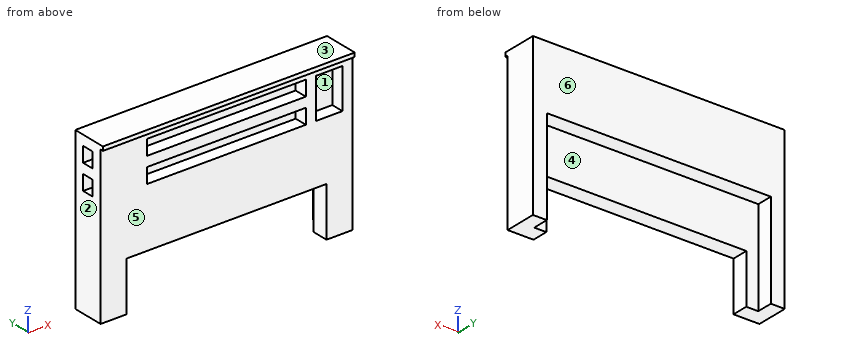
from build123d import *

# Parameters (mm, degrees)
F0_W     = 1016
F0_H     = 96.8375
F0_W_2   = 1611.3125
F0_H_2   = 25.4
F0_W_3   = 170.65625
F0_H_3   = 257.175
F1_DEPTH = 223.8375
F2_DEPTH = 101.6
F3_DEPTH = 19.05
F4_W     = 77.7875
F4_H     = 96.8375
F5_DEPTH = 190.5
F7_DEPTH = 101.6


with BuildPart() as f1:
    # F0 (on Front) → F1 (new body)
    with BuildSketch(Plane.XZ):
        Polygon((0, 698.5), (0, 0), (165.89375, 0), (165.89375, 317.5), (1445.41875, 317.5), (1445.41875, 0), (1611.3125, 0), (1611.3125, 698.5), (1547.8125, 698.5), (1377.15625, 698.5), (1313.65625, 698.5), (297.65625, 698.5), align=None)
        Polygon((0, 993.775), (0, 698.5), (297.65625, 698.5), (297.65625, 795.3375), (1313.65625, 795.3375), (1313.65625, 698.5), (1377.15625, 698.5), (1377.15625, 955.675), (1547.8125, 955.675), (1547.8125, 698.5), (1611.3125, 698.5), (1611.3125, 993.775), align=None)
        with Locations((805.65625, 907.25625)):
            Rectangle(F0_W, F0_H, mode=Mode.SUBTRACT)
        with Locations((805.65625, 746.91875)):
            Rectangle(F0_W, F0_H)
        with Locations((805.65625, 907.25625)):
            Rectangle(F0_W, F0_H)
        with Locations((805.65625, 1006.475)):
            Rectangle(F0_W_2, F0_H_2)
        with Locations((1462.484375, 827.0875)):
            Rectangle(F0_W_3, F0_H_3)
    extrude(amount=-F1_DEPTH)

    # F0 (on Front) → F2 (cut)
    with BuildSketch(Plane.XZ):
        with Locations((805.65625, 907.25625)):
            Rectangle(F0_W, F0_H)
        with Locations((805.65625, 746.91875)):
            Rectangle(F0_W, F0_H)
        with Locations((1462.484375, 827.0875)):
            Rectangle(F0_W_3, F0_H_3)
    extrude(amount=-F2_DEPTH, mode=Mode.SUBTRACT)

    # F0 (on Front) → F3 (cut)
    with BuildSketch(Plane.XZ):
        Polygon((0, 698.5), (0, 0), (165.89375, 0), (165.89375, 317.5), (1445.41875, 317.5), (1445.41875, 0), (1611.3125, 0), (1611.3125, 698.5), (1547.8125, 698.5), (1377.15625, 698.5), (1313.65625, 698.5), (297.65625, 698.5), align=None)
        Polygon((0, 993.775), (0, 698.5), (297.65625, 698.5), (297.65625, 795.3375), (1313.65625, 795.3375), (1313.65625, 698.5), (1377.15625, 698.5), (1377.15625, 955.675), (1547.8125, 955.675), (1547.8125, 698.5), (1611.3125, 698.5), (1611.3125, 993.775), align=None)
        with Locations((805.65625, 907.25625)):
            Rectangle(F0_W, F0_H, mode=Mode.SUBTRACT)
    extrude(amount=-F3_DEPTH, mode=Mode.SUBTRACT)

    # F4 (on face) → F5 (cut)
    with BuildSketch(Plane(origin=(0, 0, 0), x_dir=(0, -1, 0), z_dir=(-1, 0, 0))):
        with Locations((-121.44375, 907.25625)):
            Rectangle(F4_W, F4_H)
        with Locations((-121.44375, 746.91875)):
            Rectangle(F4_W, F4_H)
    extrude(amount=-F5_DEPTH, mode=Mode.SUBTRACT)

    # F6 (on face) → F7 (cut)
    with BuildSketch(Plane(origin=(0, 223.8375, 0), x_dir=(-1, 0, 0), z_dir=(0, 1, 0))):
        Polygon((-1522.4125, 609.6), (-1522.4125, 0), (-1445.41875, 0), (-1445.41875, 317.5), (-165.89375, 317.5), (-165.89375, 0), (-88.9, 0), (-88.9, 609.6), align=None)
    extrude(amount=-F7_DEPTH, mode=Mode.SUBTRACT)


solid = f1.part
For this review, take the finished solid that the model builds, in its own axes (mm). Face numbers are marked on the shaded views. A direction names the side the tool comes from. Coordinates: 2 decimals unless noted, no trailing zeros. Order: outer loops, then holes, each group sorted by start corner. A loop starts at its lowest first (then second) coordinate and runs counter-clockwise, first axis right, second up. Notation, with made-up numbers: (30.25, 35) - (59.25, 35) arc R25 cw to (59.25, 51) - close; hole circle Ø2 at (-0.75, -26.75). An arc over 180 degrees is marked (long way). Use one line per item in the form item = value.
Q1. For the marked faces 4, 5 and 6, list the 3-axis set-ups (+Z, -Z, +X, -X, +Y, -Y) from which the entire face can be reached by the end or side of a thin tool; tool diameter is ignored.
Checked values:
face_4 = -Z, +Y
face_5 = -Z, +X, -X, -Y
face_6 = +Z, -Z, +X, -X, +Y
Q2. For probe 1 along X at (y, z) = (68, 743); probe 2 along Z at (x, y) = (463, 75) (1 decimal); probe 3 along X at (y, z) = (101.5, 829.5), list the stretches that pass through material, from the lowest coordinate up. Write a range as from..to.
Checked values:
probe_1 = 0..297.66, 1313.66..1377.16, 1547.81..1611.31
probe_2 = 317.5..698.5, 795.3..858.8, 955.7..1019.2
probe_3 = 0..1377.16, 1547.81..1611.31
Q3. For P1, Ø1, axis at y = 51, z = 802.5, coming from the -X side; P2, Ø25, axis at x = 778.5, y = 42.5, coming from the -Z side; P3, Ø8, axis at x = 412.5, z = 603, coming from the +Y side; P4, Ø21, axis at x = 575, y = 6, coming from the -Z side (3 decimals), all flat-tipped, find the tip position at first contact; note any pin that passes through.
Checked values:
P1 = 0
P2 = 317.5
P3 = 122.24
P4 = 993.775
Q4. Consider section D-D (z = 820). Give the boundary of the cut face in (x, y).
Checked values:
outline = (0, 19.05) - (1377.16, 19.05) - (1377.16, 101.6) - (1547.81, 101.6) - (1547.81, 19.05) - (1611.31, 19.05) - (1611.31, 223.84) - (0, 223.84) - close
Q5. Consider section C-C (y = 184.5). Give the boundary of the cut face in (x, z) (1 decimal).
Checked values:
outline = (0, 0) - (88.9, 0) - (88.9, 609.6) - (1522.4, 609.6) - (1522.4, 0) - (1611.3, 0) - (1611.3, 1019.2) - (0, 1019.2) - close
Q6. Draft analysis for pull direction Z (two halves, no side actions). For the marked faces 1, 2 and 3, state which applies: +Z half, -Z half, draft (parallel to the pull), parting line (faces both ways), or undercut.
Checked values:
face_1 = undercut
face_2 = draft
face_3 = +Z half
Q7. Consider section A-A (z = 92). Give the boundary of the cut face in (x, y), then the cut area to 3 significant figures.
Checked values:
outline = (0, 19.05) - (165.89, 19.05) - (165.89, 122.24) - (88.9, 122.24) - (88.9, 223.84) - (0, 223.84) - close; (1445.42, 19.05) - (1611.31, 19.05) - (1611.31, 223.84) - (1522.41, 223.84) - (1522.41, 122.24) - (1445.42, 122.24) - close
area = 52,300 mm2
